Drawing for the job (mm, zero at the part's lowest x, y, z). A direction names the side the tool comes from. Give positions to 0.01 mm unless a question says otherwise; leave off trailing zeros. Loops run counter-clockwise (first coordinate to the right, second up) from the corner with the lowest first, then second, coordinate; pieces in that order, holes last. Notation, with made-up numbers: (17.5, 16.25) -> (51.5, 16.25) arc R21 cw to (51.5, 29.25) -> close; hole circle Ø5 at (63, 47). An arc over 180 degrees is marked (long way). Use CSV: the item, a comma, the result in double quotes. Start each with the question number.
(1) 3-axis set-ups, long thin cutter, end or side, ignore diameter. For the marked faces 1 and 2: which of +Z, -Z, +X, -X, +Y, -Y reach the whole face in a straight line?
(2) Cut at A-A on y = 22.5. Write the cut outline in (x, z), then the cut area to 3 significant figures.
(3) Drill centre lines: probe 1 along Y at (x, z) = (38, 6.5); probe 2 along X at (y, z) = (23.5, 7.75); probe 3 along X at (y, z) = (47.5, 6.75). Where is each one in solid material? Low to high.
(4) Flat gauge pins, fed straight in: pin 1 (7 mm diameter, centred on y = 5.29, z = 6.5, fed in from +X); pin 2 (1.2 mm diameter, centred on y = 44.5, z = 7, fed in from +X); pin 3 (1 mm diameter, centred on x = 1.5, z = 7.5, fed in from +Y); pin 4 (1.8 mm diameter, centred on x = 37.5, z = 9.5, fed in from +Y). Where does each tip first touch, or does it go through?
(5) Pull direction Y, two halves, no side cores. Call the marked faces 3, 4 and 5: pulls with the +Y half, pulls with the -Y half, needs draft (parallel to the pull), parting line crosses it, or undercut.
(6) Cut at D-D on z = 11. Write the cut outline in (x, y), then the cut area to 3 significant figures.
(7) Cut at C-C on z = 1.25. Write the cut outline in (x, y), then the cut area to 3 significant figures.
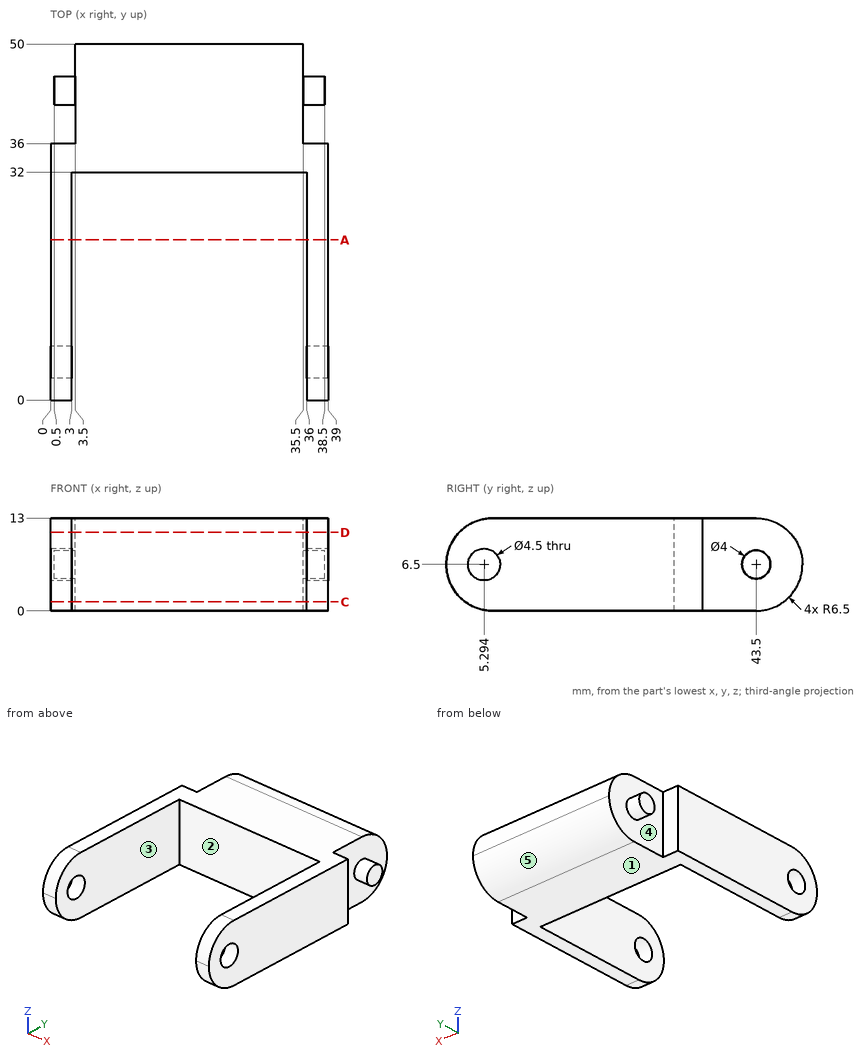
Check result:
1,face 1,"-Z, +X, -X, +Y, -Y"
1,face 2,"+Z, -Z, -Y"
2,outline,"(0, 0) -> (3, 0) -> (3, 13) -> (0, 13) -> close; (36, 0) -> (39, 0) -> (39, 13) -> (36, 13) -> close"
2,area,"78.0 mm²"
3,probe 1,"0 to 3.04, 7.54 to 36, 41.5 to 45.5"
3,probe 2,"0 to 3, 36 to 39"
3,probe 3,"3.5 to 35.5"
4,pin 1,"x = 39"
4,pin 2,"x = 38.5"
4,pin 3,"y = 45.44"
4,pin 4,"y = 36"
5,face 3,"needs draft"
5,face 4,"undercut"
5,face 5,"pulls with the +Y half"
6,outline,"(0, 1.81) -> (3, 1.81) -> (3, 32) -> (36, 32) -> (36, 1.81) -> (39, 1.81) -> (39, 36) -> (35.5, 36) -> (35.5, 48.19) -> (3.5, 48.19) -> (3.5, 36) -> (0, 36) -> close"
6,area,"727 mm²"
7,outline,"(0, 2.67) -> (3, 2.67) -> (3, 32) -> (36, 32) -> (36, 2.67) -> (39, 2.67) -> (39, 36) -> (35.5, 36) -> (35.5, 47.33) -> (3.5, 47.33) -> (3.5, 36) -> (0, 36) -> close"
7,area,"695 mm²"
